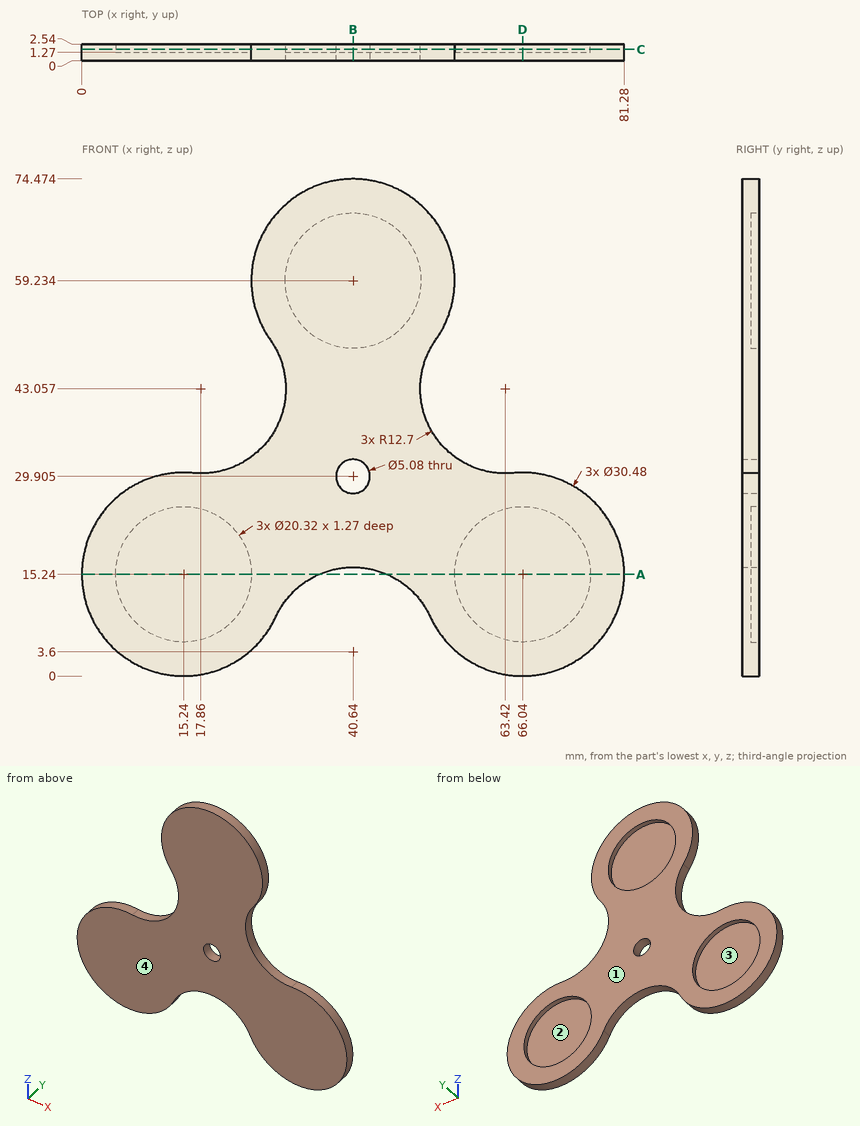
For this review, use the dimensioned drawing (mm, ordinates from the lowest corner) and the shaded views. A direction names the side the tool comes from. Give positions to 0.01 mm unless a question says otherwise; leave off trailing zeros. Write each loop counter-clockwise with the first axis right and the second up, starting at its lowest first coordinate (ties: lowest second). Pieces come first, ordered by that corner, then holes.
(1) Consider section C-C, the plane y = 1.75. Give the boundary of the cut face in (x, z) (1 decimal), and give its area (3 significant figures).
(2) To check wall thickness, follow L1, parallel to X at y = 1.9, z = 8.5; L2, parallel to Z at x = 15.24, y = 2; L3, parallel to Z at x = 21.5, y = 1.85 (1 decimal). State the ranges of each line that lie inside material, in increasing order.
(3) For P1, Ø18.5, axis at x = 15.24, z = 15.24, coming from the -Y side; P2, Ø6, axis at x = 68.5, z = 15, coming from the +Y side; P3, Ø3, axis at x = 40.64, z = 29.9, coming from the -Y side, all flat-tipped, find the tip position at first contact; note any pin that passes through.
(4) Consider section B-B, the plane x = 40.64. Give the boundary of the cut face in (y, z) (1 decimal).
(5) Consider section A-A, the plane z = 15.24. Give the boundary of the cut face in (x, y).
(6) Consider section D-D, the plane x = 66.04. Give the boundary of the cut face in (y, z).
(7) Tool access review of the marked faces 1 and 2: name each direction out of +Z, -Z, +X, -X, +Y, -Y from which nothing blocks a thin tool from reaching the whole face with its end or side.
(8) The part is to be moulded in two halves that separate along Z. For the marked faces 3 and 4, say which applies: released by +Z, released by -Z, zero draft, split by the parting line, or undercut.
Returned:
1. outline: (16.7, 30.4) arc R15.2 ccw (long way) to (29.1, 8.9) arc R12.7 cw to (52.2, 8.9) arc R15.2 ccw (long way) to (64.6, 30.4) arc R12.7 cw to (53.1, 50.4) arc R15.2 ccw (long way) to (28.2, 50.4) arc R12.7 cw to start; hole circle Ø20.3 at (15.2, 15.2); hole circle Ø20.3 at (40.6, 59.2); hole circle Ø5.1 at (40.6, 29.9); hole circle Ø20.3 at (66, 15.2)
1. area: 1,980 mm2
2. L1: x = 1.57 to 7.64, 22.84 to 28.91, 52.37 to 58.44, 73.64 to 79.71
2. L2: z = 0 to 5.08, 25.4 to 30.48
2. L3: z = 1.3 to 7.2, 23.2 to 30.9
3. P1: stops at y = 0
3. P2: stops at y = 1.27
3. P3: passes through
4. outline: (0, 16.3) - (2.5, 16.3) - (2.5, 27.4) - (0, 27.4) - close; (0, 32.4) - (2.5, 32.4) - (2.5, 49.1) - (1.3, 49.1) - (1.3, 69.4) - (2.5, 69.4) - (2.5, 74.5) - (0, 74.5) - close
5. outline: (0, 0) - (35.56, 0) - (35.56, 2.54) - (25.4, 2.54) - (25.4, 1.27) - (5.08, 1.27) - (5.08, 2.54) - (0, 2.54) - close; (45.72, 0) - (81.28, 0) - (81.28, 2.54) - (76.2, 2.54) - (76.2, 1.27) - (55.88, 1.27) - (55.88, 2.54) - (45.72, 2.54) - close
6. outline: (0, 0) - (2.54, 0) - (2.54, 5.08) - (1.27, 5.08) - (1.27, 25.4) - (2.54, 25.4) - (2.54, 30.48) - (0, 30.48) - close
7. face 1: +Z, -Z, +X, -X, +Y
7. face 2: +Y
8. face 3: undercut
8. face 4: zero draft
